Here's how the part is built. I have some questions about the finished solid (model axes, mm). Give positions to 0.01 mm unless a question says otherwise; leave off trailing zeros. Write each loop counter-clockwise with the first axis right and the second up, starting at its lowest first coordinate (ties: lowest second). Pieces come first, ordered by that corner, then holes. Notation, with made-up numbers: M -25.5,20.5 L 0.5,20.5 A6 cw 0.5,25.5 Z; hole C -6,-23.75 d7. An arc over 180 degrees is marked long. Answer as CSV lines item,"result". Start each with the question number.
Q1. Suppose I cut it at A-A (x = 12). Write out the boundary of the cut face in (y, z), then the cut area to 3 significant figures.
Q2. If I drill on line 1 along Y through (x, z) = (0, 0.4); line 2 along Y through (x, z) = (-12, 1.55); line 3 along Y through (x, z) = (-33, 1.25), over which ranges is the centre line in solid material (lowest first)?
Q3. Suppose I cut it at C-C (x = 40). Write out the boundary of the cut face in (y, z).
Q4. For pin 1 (1 mm diameter, centred on y = 4, z = 0.5, fed in from -X); pin 2 (1 mm diameter, centred on y = 5, z = 1.5, fed in from -X); pin 3 (0.6 mm diameter, centred on x = -25.5, z = 1, fed in from -Y); pin 4 (2.5 mm diameter, centred on x = 12, y = -12, fed in from -Z), each with a flat end and sliding along its axis, tell me the tip position at first contact or that it passes through.
Q5. Suppose I cut it at B-B (z = 1.7). Count the separate pieces of the cut face and the enclosed holes in it, then the cut area to 3 significant figures.
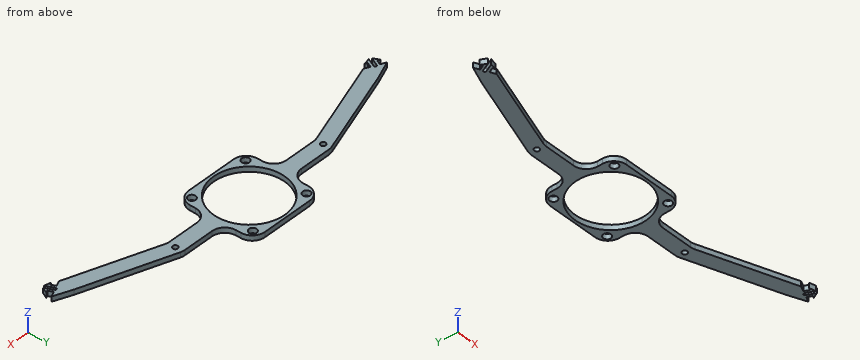
```python
from build123d import *

# Parameters (mm, degrees)
F0_R     = 1.5
F0_R_2   = 1
F1_DEPTH = 2
F2_R     = 5


with BuildPart() as f1:
    # F0 (on Top) → F1 (new body)
    with BuildSketch(Plane.XY):
        with BuildLine():
            ThreePointArc((13.5, -12), (12, -10.5), (10.5, -12))
            ThreePointArc((10.5, -12), (12, -13.5), (13.5, -12))
        make_face()
        with BuildLine():
            Line((15, 3), (15, 15))
            Line((15, 15), (-15, 15))
            Line((-15, 15), (-15, 3))
            Line((-15, 3), (-33, 3))
            Line((-33, 3), (-68, -9))
            Line((-68, -9), (-74.892196, -11.786116))
            Line((-74.892196, -11.786116), (-72.80556, -12.759131))
            Line((-72.80556, -12.759131), (-73.650796, -14.571746))
            Line((-73.650796, -14.571746), (-74.581683, -14.137667))
            Line((-74.581683, -14.137667), (-73.422492, -16.448347))
            Line((-73.422492, -16.448347), (-71.899252, -13.181749))
            ThreePointArc((-71.899252, -13.181749), (-71.234789, -12.939904), (-70.992944, -13.604367))
            Line((-70.992944, -13.604367), (-72.516184, -16.870966))
            Line((-72.516184, -16.870966), (-70.000987, -16.27368))
            Line((-70.000987, -16.27368), (-70.931873, -15.839601))
            Line((-70.931873, -15.839601), (-70.086637, -14.026985))
            Line((-70.086637, -14.026985), (-68, -15))
            Line((-68, -15), (-33, -3))
            Line((-33, -3), (-15, -3))
            Line((-15, -3), (-15, -15))
            Line((-15, -15), (15, -15))
            Line((15, -15), (15, -3))
            Line((15, -3), (33, -3))
            Line((33, -3), (68, -15))
            Line((68, -15), (70.086637, -14.026985))
            Line((70.086637, -14.026985), (70.931873, -15.839601))
            Line((70.931873, -15.839601), (70.000987, -16.27368))
            Line((70.000987, -16.27368), (72.516184, -16.870966))
            Line((72.516184, -16.870966), (70.992944, -13.604367))
            ThreePointArc((70.992944, -13.604367), (71.234789, -12.939904), (71.899252, -13.181749))
            Line((71.899252, -13.181749), (73.422492, -16.448347))
            Line((73.422492, -16.448347), (74.581683, -14.137667))
            Line((74.581683, -14.137667), (73.650796, -14.571746))
            Line((73.650796, -14.571746), (72.80556, -12.759131))
            Line((72.80556, -12.759131), (74.892196, -11.786116))
            Line((74.892196, -11.786116), (68, -9))
            Line((68, -9), (33, 3))
            Line((33, 3), (15, 3))
        make_face()
        with Locations((-12, -12)):
            Circle(F0_R, mode=Mode.SUBTRACT)
        with BuildLine():
            ThreePointArc((13.5, -12), (12, -13.5), (10.5, -12))
            ThreePointArc((10.5, -12), (12, -10.5), (13.5, -12))
        make_face(mode=Mode.SUBTRACT)
        with Locations((-33, 0)):
            Circle(F0_R_2, mode=Mode.SUBTRACT)
        with Locations((-12, 12)):
            Circle(F0_R, mode=Mode.SUBTRACT)
        with BuildLine():
            ThreePointArc((14, 0), (12.185143, -6.893641), (7.211103, -12))
            ThreePointArc((7.211103, -12), (-12.185143, 6.893641), (14, 0))
        make_face(mode=Mode.SUBTRACT)
        with Locations((33, 0)):
            Circle(F0_R_2, mode=Mode.SUBTRACT)
        with Locations((12, 12)):
            Circle(F0_R, mode=Mode.SUBTRACT)
    extrude(amount=F1_DEPTH)

    # F2
    f2_edges = [f1.edges().sort_by_distance(p)[0] for p in [
        (33, -3, 1),
        (33, 3, 1),
        (15, 3, 1),
        (15, -3, 1),
        (15, -15, 1),
        (15, 15, 1),
        (-15, 15, 1),
        (-33, 3, 1),
        (-15, -15, 1),
        (-33, -3, 1),
        (-15, -3, 1),
        (-15, 3, 1),
    ]]
    fillet(f2_edges, radius=F2_R)


solid = f1.part
```
Resolved:
1,outline,"M -14.58,0 L -13.5,0 L -13.5,2 L -14.58,2 Z; M -10.5,0 L -7.21,0 L -7.21,2 L -10.5,2 Z; M 7.21,0 L 10.5,0 L 10.5,2 L 7.21,2 Z; M 13.5,0 L 14.58,0 L 14.58,2 L 13.5,2 Z"
1,area,"17.5 mm^2"
2,line 1,"-15 to -14, 14 to 15"
2,line 2,"-14.58 to -13.5, -10.5 to -7.21, 7.21 to 10.5, 13.5 to 14.58"
2,line 3,"-3.07 to -1, 1 to 2.93"
3,outline,"M -5.4,0 L 0.6,0 L 0.6,2 L -5.4,2 Z"
4,pin 1,"x = -17.82"
4,pin 2,"x = -16.43"
4,pin 3,"y = -3"
4,pin 4,"through"
5,separate pieces,"1"
5,enclosed holes,"7"
5,area,"941 mm^2"
